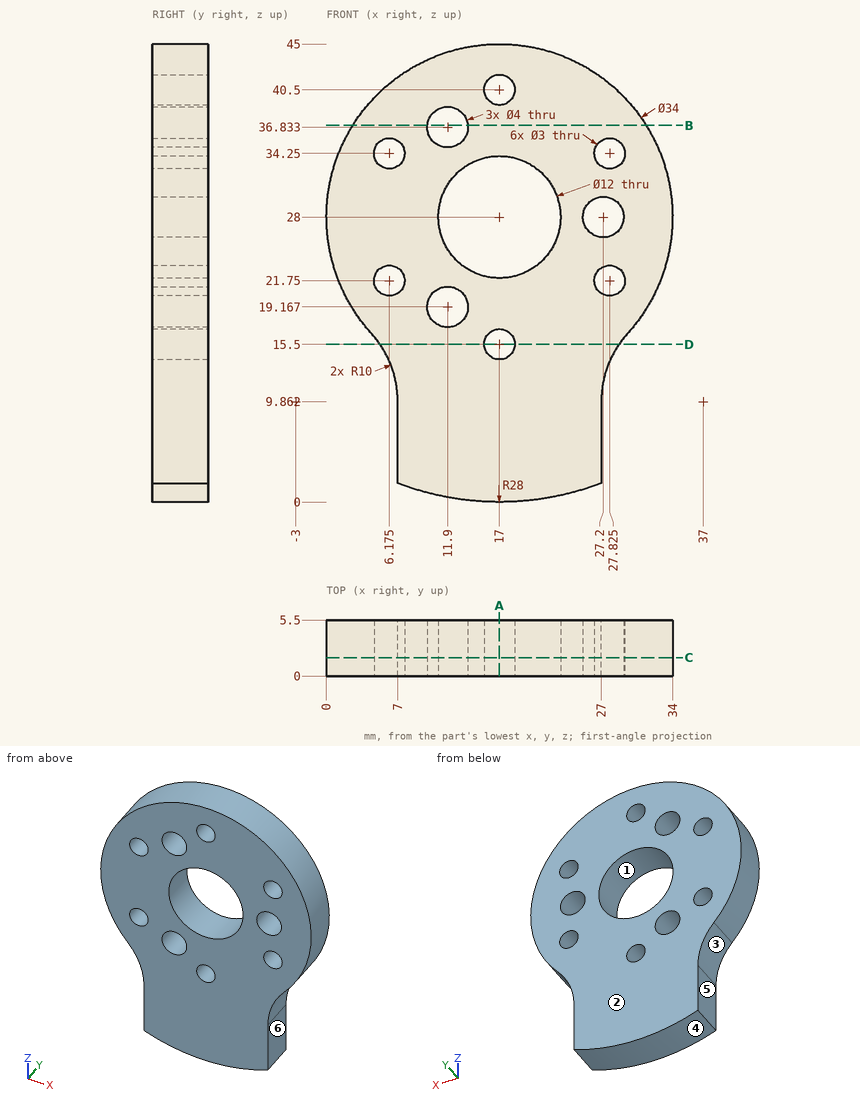
Can you work these out from the drawing? Everything is in mm from the part's minimum corner. A direction names the side the tool comes from. Coordinates: 2 decimals unless noted, no trailing zeros. Loops run counter-clockwise (first coordinate to the right, second up) from the corner with the lowest first, then second, coordinate; pieces in that order, holes last. Notation, with made-up numbers: M 54,87 L 87,87 A26 cw 87,121 Z; hole C 82,-2 d4. An arc over 180 degrees is marked long. Put each result on its own line as item: value. Start each with the question number.
(1) Suppose I cut it at C-C on y = 1.8. Count the separate pieces of the cut face and the enclosed holes in it, then the cut area to 3 significant figures.
(2) Suppose I cut it at A-A on x = 17. Please give me the cut outline in (y, z).
(3) I need wall thicknesses on line 1 (X direction, y = 2.5, z = 28); line 2 (Z direction, x = 16, y = 2.3) (1 decimal); line 3 (X direction, y = 1.95, z = 8.5). Which ranges of each line are inside material? Lowest first, please. Write a range as from..to.
(4) Thinking about a two-plate mould opening in Z: for the marked faces 1, 2 and 3, which applies, pulls with the +Z half, pulls with the -Z half, needs draft (parallel to the pull), parting line crosses it, or undercut?
(5) For the marked faces 4, 5 and 6, which set-ups out of +Z, -Z, +X, -X, +Y, -Y let a thin tool reach every point of the face, with its end or its side?
(6) Will these pins go through, and if not, where does the flat tip stop? P1, Ø1.6, axis at y = 2.5, z = 7.5, coming from the -X side; P2, Ø1.5, axis at y = 1, z = 20.5, coming from the -X side; P3, Ø1.5, axis at x = 15, y = 3.5, coming from the -Z side.
(7) Suppose I cut it at D-D on z = 15.5. Please give me the cut outline in (x, y), then the cut area to 3 significant figures.
(8) Suppose I cut it at B-B on z = 37. Please give me the cut outline in (x, y), then the cut area to 3 significant figures.
Solutions:
1. separate pieces: 1
1. enclosed holes: 10
1. area: 948 mm2
2. outline: M 0,0 L 5.5,0 L 5.5,14 L 0,14 Z; M 0,17 L 5.5,17 L 5.5,22 L 0,22 Z; M 0,34 L 5.5,34 L 5.5,39 L 0,39 Z; M 0,42 L 5.5,42 L 5.5,45 L 0,45 Z
3. line 1: x = 0..11, 23..25.2, 29.2..34
3. line 2: z = 0..14.4, 16.6..22.1, 33.9..39.4, 41.6..45
3. line 3: x = 7..27
4. face 1: undercut
4. face 2: needs draft
4. face 3: pulls with the -Z half
5. face 4: -Z, +Y, -Y
5. face 5: -Z, -X, +Y, -Y
5. face 6: -Z, +X, +Y, -Y
6. P1: stops at x = 7
6. P2: stops at x = 1.4
6. P3: stops at z = 0.03
7. outline: M 5.26,0 L 15.5,0 L 15.5,5.5 L 5.26,5.5 Z; M 18.5,0 L 28.74,0 L 28.74,5.5 L 18.5,5.5 Z
7. area: 113 mm2
8. outline: M 2.58,0 L 9.91,0 L 9.91,5.5 L 2.58,5.5 Z; M 13.89,0 L 31.42,0 L 31.42,5.5 L 13.89,5.5 Z
8. area: 137 mm2
